Input: part model. Units: mm. Frame: model coordinates. A direction names the side the tool comes from. Give positions to 0.01 mm unless a question says otherwise; leave off trailing zeros. Order: outer loops, then holes, each group sorted by start corner. A loop starts at its lowest first (then second) coordinate and runs counter-clockwise, first axis right, second up. Notation, with made-up numbers: (54.5, 26.5) - (74.5, 26.5) arc R36 ccw to (74.5, 61.5) - close; hole circle Ø10 at (34, 41.5). An arc over 180 degrees is marked (long way). Answer in a Markdown table with one row per item. Add a question column.
1. Access query for faces 1 (the face through (70, 0, -3)), 2 (the face through (292.48, -2.44, 0.54)), 3 (the face through (191.159, -3.905, 0.867)). Directions: +Z, -Z, +X, -X, +Y, -Y. A direction counts if a zero-diameter tool reaches every point of the face in a straight line with its end or side. Return the directions, or none.
2. Section query A-A on z = 0. Return loops of the section in (x, y), and give its area (3 significant figures).
3. Contact query for flat-ended pins moving along their axis: pin 1 (3 mm diameter, centred on x = 75.5, y = 3, fed in from -Z); pin 2 (3 mm diameter, centred on x = 79, z = 1.5, fed in from -Y); pin 3 (1.5 mm diameter, centred on y = 3, z = 2.5, fed in from +X). Output: stop coordinate, or through.
4. Ray query, line 1 (X direction, y = -2.75, z = -2.5); line 2 (Z direction, x = 133, y = -0.25); line 3 (Y direction, x = 95, z = 0.25). Return the intervals inside material, ascending. Write a range as [from, to].
5. Section query B-B on x = 70.5. Return loops of the section in (y, z), and give its area (3 significant figures).
6. Section query C-C on x = 260.5. Return loops of the section in (y, z), and give its area (3 significant figures).
Autodesk Inventor part; units mm, degrees
ref_plane "YZ Plane" through (0, 0, 0) normal (1, 0, 0) x (0, 1, 0)
ref_plane "XZ Plane" through (0, 0, 0) normal (0, 1, 0) x (-1, 0, 0)
ref_plane "XY Plane" through (0, 0, 0) normal (0, 0, 1) x (1, 0, 0)
sketch "Sketch1" plane through (0, 0, 0) normal (1, 0, 0) x (0, 1, 0)
  circle A0 centre (0, 0) radius 6.35
  dimension "d0" = 12.7
extrude "Extrusion1" add sketch "Sketch1" along normal blind 304.8
sketch "Sketch2" plane through (304.8, 0, 0) normal (1, 0, 0) x (0, 0, -1)
  circle A0 centre (0, 0) radius 4.7625
  circle A1 centre (0, 0) radius 6.35
  dimension "d3" = 9.525
extrude "Extrusion2" cut sketch "Sketch2" against normal blind 385.2875
sketch "Sketch3" plane through (304.8, 0, 0) normal (1, 0, 0) x (0, 0, -1)
  circle A0 centre (0, 0) radius 4
  circle A1 centre (0, 0) radius 4.7625
  dimension "d6" = 8
extrude "Extrusion3" cut sketch "Sketch3" against normal blind 369.4125
sketch "Sketch4" plane through (304.8, 0, 0) normal (1, 0, 0) x (0, 0, -1)
  circle A0 centre (0, 0) radius 3
  circle A1 centre (0, 0) radius 4
  dimension "d9" = 6
extrude "Extrusion4" cut sketch "Sketch4" against normal blind 25
sketch "Sketch5" plane through (0, 0, 0) normal (-1, 0, 0) x (0, 0, 1)
  circle A0 centre (0, 0) radius 2.5
  circle A1 centre (0, 0) radius 4
  dimension "d12" = 5
extrude "Extrusion5" cut sketch "Sketch5" against normal blind 25
sketch "Sketch7" plane through (304.8, 0, 0) normal (1, 0, 0) x (0, 0, -1)
  circle A0 centre (0, 0) radius 2.5
  circle A1 centre (0, 0) radius 3
  dimension "d15" = 5
extrude "Extrusion6" cut sketch "Sketch7" against normal blind 25
sketch "Sketch8" plane through (0, 0, 0) normal (-1, 0, 0) x (0, 0, 1)
  circle A0 centre (0, 0) radius 4
  dimension "d18" = 8
extrude "Extrusion7" cut sketch "Sketch8" against normal blind 100
sketch "Sketch9" plane through (100, 0, 0) normal (-1, 0, 0) x (0, 0, 1)
  circle A0 centre (0, 0) radius 4
extrude "Extrusion8" add sketch "Sketch9" along normal blind 60
sketch "Sketch10" plane through (40, 0, 0) normal (-1, 0, 0) x (0, 0, 1)
  circle A0 centre (0, 0) radius 3
  circle A1 centre (0, 0) radius 4
  dimension "d23" = 6
extrude "Extrusion9" cut sketch "Sketch10" against normal blind 60
properties part number "Lead_Shaft" material "Steel, Carbon"
Answer:
| question | item | result |
|---|---|---|
| 1 | face 1 | -X |
| 1 | face 2 | +X |
| 1 | face 3 | +X, -X |
| 2 | outline | (40, -3) - (100, -3) - (100, -4) - (279.8, -4) - (279.8, -2.5) - (304.8, -2.5) - (304.8, 2.5) - (279.8, 2.5) - (279.8, 4) - (100, 4) - (100, 3) - (40, 3) - close |
| 2 | area | 1,920 mm² |
| 3 | pin 1 | stops at z = -2.6 |
| 3 | pin 2 | stops at y = -3 |
| 3 | pin 3 | stops at x = 279.8 |
| 4 | line 1 | x = [100, 279.8] |
| 4 | line 2 | z = [-3.99, 3.99] |
| 4 | line 3 | y = [-2.99, 2.99] |
| 5 | outline | circle Ø6 at (0, 0) |
| 5 | area | 28.3 mm² |
| 6 | outline | circle Ø8 at (0, 0) |
| 6 | area | 50.3 mm² |
